Build history of the part. All positions in model axes, mm. A direction names the side the tool comes from. Coordinates: 2 decimals unless noted, no trailing zeros. Loops run counter-clockwise (first coordinate to the right, second up) from the corner with the lowest first, then second, coordinate; pieces in that order, holes last. Notation, with made-up numbers: (-9.75, 49) - (44.25, 49) arc R32 cw to (44.25, 87) - close; hole circle Ø6 at (49, 53.5). An arc over 180 degrees is marked (long way). One line per item, written item: value.
Autodesk Inventor part; units mm, degrees
ref_plane "YZ Plane" through (0, 0, 0) normal (1, 0, 0) x (0, 1, 0)
ref_plane "XZ Plane" through (0, 0, 0) normal (0, 1, 0) x (-1, 0, 0)
ref_plane "XY Plane" through (0, 0, 0) normal (0, 0, 1) x (1, 0, 0)
sketch "Sketch1" plane through (0, 0, 0) normal (0, 1, 0) x (-1, 0, 0)
  line L0 (0, 0) -> (-50.8, 0)
  line L1 (-50.8, 0) -> (-50.8, -88.9)
  line L2 (-50.8, -88.9) -> (0, -88.9)
  line L3 (0, -88.9) -> (0, 0)
  dimension "d0" = 50.8
  dimension "d1" = 88.9
extrude "Extrusion1" add sketch "Sketch1" along normal blind 12.7
sketch "Sketch2" plane through (0, 12.7, 0) normal (0, 1, 0) x (1, 0, 0)
  line L0 (50.8, 0) -> (50.8, 88.9)
  line L1 (50.8, 88.9) -> (0, 88.9)
  line L2 (0, 88.9) -> (0, 0)
  line L3 (6.35, 88.9) -> (44.45, 88.9)
  line L4 (44.45, 88.9) -> (44.45, 69.85)
  line L5 (44.45, 69.85) -> (6.35, 69.85)
  line L6 (6.35, 69.85) -> (6.35, 88.9)
  line L7 (6.35, 79.375) -> (0, 79.375) construction
  line L8 (44.45, 79.375) -> (50.8, 79.375) construction
  circle A0 centre (25.4, 69.85) radius 19.05
  dimension "d4" = 19.05
  dimension "d5" = 6.35
extrude "Extrusion2" add sketch "Sketch2" along normal blind 12.7
sketch "Sketch3" plane through (0, 25.4, 0) normal (0, 1, 0) x (1, 0, 0)
  arc A0 (6.35, 69.85) -> (44.45, 69.85) centre (25.4, 69.85) ccw
  circle A1 centre (25.4, 69.85) radius 12.7
  point P0 (0, 0)
  dimension "d8" = 25.4
extrude "Extrusion3" add sketch "Sketch3" along normal blind 12.7
fillet "Fillet2" radius 4.7625 5 edges at (50.8, 6.35, 0) (0, 6.35, 0) (6.35, 12.7, -79.375) (44.45, 12.7, -79.375) (25.4, 12.7, -50.8)
chamfer "Chamfer1" distance 6.35 distance2 3.175 3 edges at (44.45, 25.4, -79.375) (25.4, 25.4, -50.8) (6.35, 25.4, -79.375) measured on face at (24.8897, 25.4, -86.7525)
properties part number "Fillet Chamfer Complete"
Item 1: Probe probe 1 along Y at (x, z) = (7, -39); probe 2 along Y at (x, z) = (11.5, -52); probe 3 along Z at (x, y) = (4.5, 12). List the from-to ranges inside material, lowest first. Write a range as from..to.
Check result:
probe 1: y = 0..12.7
probe 2: y = 0..12.85
probe 3: z = -88.9..-0.01
Item 2: Cut at D-D, the plane y = 21. Write the cut outline in (x, z), then the cut area to 3 significant figures.
Check result:
outline: (6.35, -88.9) - (44.45, -88.9) - (44.45, -69.85) arc R19.05 ccw to (6.35, -69.85) - close
area: 1,300 mm^2
Item 3: Drop flat-ended pins along their axis: P1, Ø8, axis at y = 18.5, z = -69.5, coming from the -X side; P2, Ø3, axis at y = 15, z = -54.5, coming from the -X side; P3, Ø4, axis at y = 20, z = -79, coming from the -X side; P4, Ø1, axis at x = 39.5, y = 25.5, coming from the +Z side. Give the stop position or say it passes through.
Check result:
P1: stops at x = 5.32
P2: stops at x = 10.46
P3: stops at x = 6.35
P4: passes through
Item 4: Tool access for faces 1 (the face through (25.819, 19.811, -50.805)), 2 (the face through (6.35, 20, -79)), 3 (the face through (25, 25.4, -84)): list every direction of +Z, -Z, +X, -X, +Y, -Y with a clear straight run to the whole face (end or side of a thin tool).
Check result:
face 1: +Z, +Y
face 2: +Z, -Z, -X, +Y
face 3: -Z, +Y
Item 5: Cut at C-C, the plane z = -38.5. Write the cut outline in (x, y).
Check result:
outline: (0, 0) - (50.8, 0) - (50.8, 12.7) - (0, 12.7) - close
Item 6: Pull direction Z, two halves, no side cores. Call faces 4 (the face through (1.36, 6.44, -1.43)), 5 (the face through (26, 13, -88.9)), 6 (the face through (41.3, 23.8, -79.5)): released by +Z, released by -Z, zero draft, split by the parting line, or undercut.
Check result:
face 4: released by +Z
face 5: released by -Z
face 6: zero draft
Item 7: Cut at B-B, the plane y = 35. Write the cut outline in (x, z).
Check result:
outline: circle Ø25.4 at (25.4, -69.85)
